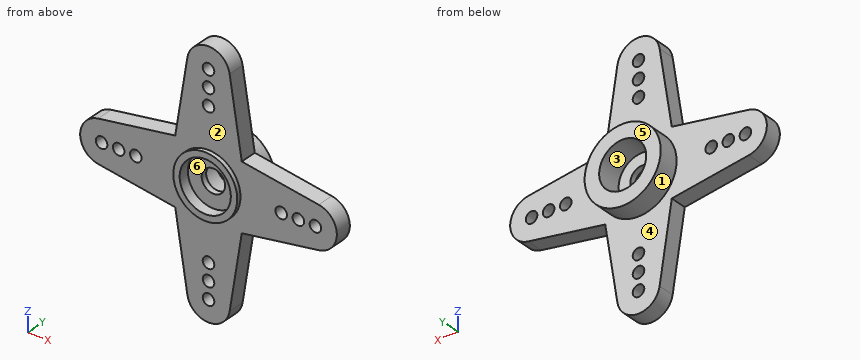
Autodesk Inventor part; units mm, degrees
ref_plane "YZ Plane" through (0, 0, 0) normal (1, 0, 0) x (0, 1, 0)
ref_plane "XZ Plane" through (0, 0, 0) normal (0, 1, 0) x (-1, 0, 0)
ref_plane "XY Plane" through (0, 0, 0) normal (0, 0, 1) x (1, 0, 0)
sketch "Sketch1" plane through (0, 0, 0) normal (0, 1, 0) x (-1, 0, 0)
  circle A0 centre (0, 0) radius 3.74
  circle A1 centre (0, 0) radius 4.45
  circle A2 centre (0, 0) radius 8.5
  circle A3 centre (0, 0) radius 10.5
  circle A4 centre (0, 0) radius 12.5
  circle A5 centre (12.5, 0) radius 2.5
  line L0 (0.6942, 4.3955) -> (12.89, 2.4694)
  line L1 (0.6942, -4.3955) -> (12.89, -2.4694)
  circle A6 centre (12.5, 0) radius 0.675
  circle A7 centre (10.5, -0.0001) radius 0.675
  circle A8 centre (8.5, 0.0004) radius 0.675
  line L2 (-4.3955, 0.6942) -> (-2.4694, 12.89)
  circle A9 centre (0, 12.5) radius 2.5
  circle A10 centre (0, 12.5) radius 0.675
  circle A11 centre (0.0001, 10.5) radius 0.675
  circle A12 centre (-0.0004, 8.5) radius 0.675
  line L3 (4.3955, 0.6942) -> (2.4694, 12.89)
  line L4 (-0.6942, -4.3955) -> (-12.89, -2.4694)
  circle A13 centre (-12.5, 0) radius 2.5
  circle A14 centre (-12.5, 0) radius 0.675
  circle A15 centre (-10.5, 0.0001) radius 0.675
  circle A16 centre (-8.5, -0.0004) radius 0.675
  line L5 (-0.6942, 4.3955) -> (-12.89, 2.4694)
  line L6 (4.3955, -0.6942) -> (2.4694, -12.89)
  circle A17 centre (0, -12.5) radius 2.5
  circle A18 centre (0, -12.5) radius 0.675
  circle A19 centre (-0.0001, -10.5) radius 0.675
  circle A20 centre (0.0004, -8.5) radius 0.675
  line L7 (-4.3955, -0.6942) -> (-2.4694, -12.89)
  point P0 (3.8907, 3.8907)
  point P1 (-3.8907, 3.8907)
  point P2 (-3.8907, -3.8907)
  point P3 (3.8907, -3.8907)
  dimension "d5" = 17
  dimension "d6" = 21
  dimension "d7" = 25
  dimension "d3" = 7.48
  dimension "d4" = 8.9
  dimension "d8" = 5
  dimension "d11" = 1.35
  dimension "d12" = 1.35
  dimension "d13" = 1.35
  dimension "d16" = 360
extrude "Extrusion1" add sketch "Sketch1" along normal blind 2 contours A1 L3 L0 A2 A8 L1 L6 | A1 L0 L3 | L6 L1 A1 | A1 L5 L2 A2 A12 L3 L0 | L1 L6 A2 A20 L7 L4 A1 | A1 L2 L5 | L0 A3 A5 A7 L1 A2 A8 | A2 A12 L2 A3 A9 A11 L3 | L4 L7 A1 | L6 A3 A17 A19 L7 A2 A20 | A1 L7 L4 A2 A16 L5 L2 | L0 A4 A5 A3 | A3 A9 A4 L3 | A3 A5 A4 L1 | L6 A4 A17 A3 | A2 A16 L4 A3 A13 A15 L5 | A5 A4 A6 A3 A7 | A3 A7 A5 | L0 A5 A4 | A9 A11 A3 | A3 A11 A9 A4 A10 | A4 A9 L3 | A5 A7 A3 | A4 A5 L1 | A17 A4 A18 A3 A19 | A3 A19 A17 | L6 A17 A4 | L2 A4 A9 A3 | A3 A13 A4 L5 | A5 A4 A6 | A4 A10 A9 | L4 A4 A13 A3 | A3 A17 A4 L7 | A17 A4 A18 | A3 A11 A9 | L2 A9 A4 | A13 A15 A3 | A3 A15 A13 A4 A14 | A4 A13 L5 | A3 A15 A13 | L4 A13 A4 | A17 A19 A3 | A4 A17 L7 | A4 A14 A13 picked at (10.283, 0.9379) picked at (0.938, 10.2831) picked at (10.2831, -0.938) picked at (0.9379, -10.283) picked at (-0.9379, 10.283) picked at (-10.2831, 0.938) picked at (-10.283, -0.9379) picked at (-0.938, -10.2831)
extrude "Extrusion2" add sketch "Sketch1" along normal blind 4.44 contours A1
ref_plane "Work Plane2" through (0, 1.44, 0) normal (0, 1, 0) x (1, 0, 0)
sketch "Sketch3" plane through (0, 1.44, 0) normal (0, 1, 0) x (1, 0, 0)
  circle A0 centre (0, 0) radius 1.37
  circle A1 centre (0, 0) radius 2.75
  circle A2 centre (0, 0) radius 2.99
  circle A3 centre (0, 0) radius 3.74
  dimension "d32" = 2.74
  dimension "d33" = 5.5
  dimension "d34" = 5.98
  dimension "d35" = 7.48
extrude "Extrusion6" add sketch "Sketch3" along normal blind 3 and the other way blind 1.94 contours A3
extrude "Extrusion7" add sketch "Sketch3" along normal blind 3 and the other way blind 0.69 contours A2
extrude "Extrusion8" add sketch "Sketch3" against normal blind 0.69 contours A1
properties part number "Standard Servo Horn - White Cross"
Can you work these out from the model? Positions are in its coordinate system, mm. Face numbers are marked on the shaded views. A direction names the side the tool comes from. Give positions to 0.01 mm unless a question says otherwise; leave off trailing zeros. Loops run counter-clockwise (first coordinate to the right, second up) from the corner with the lowest first, then second, coordinate; pieces in that order, holes last. Notation, with made-up numbers: M 80,35 L 138,35 A11 ccw 138,51 Z; hole C 34.5,-18 d3. An arc over 180 degrees is marked long. Use CSV: the item, a comma, the result in double quotes. Start each with the question number.
1. Imagine slicing it at A-A, the plane z = 10.5. Write out the boundary of the cut face in (x, y), plus the area to 3 significant figures.
2. Imagine slicing it at B-B, the plane x = 12.5. Write out the boundary of the cut face in (y, z) (3 decimals).
3. If we mould it in two halves opening along X, with no side actions, what happens to the marked faces 1, 2 and 3? For each: released by +X, released by -X, zero draft, split by the parting line, or undercut.
4. For P1, Ø1.8, axis at x = 0, z = -12.5, coming from the -Y side; P2, Ø1.8, axis at x = 0, z = 8.5, coming from the +Y side; P3, Ø9, axis at x = -3.5, z = 6, coming from the +Y side, each with a flat end and sliding along its axis, tell me the tip position at first contact or that it passes through.
5. Imagine slicing it at D-D, the plane x = 0. Count the separate pieces of the cut face and the enclosed holes in it, plus the area to 3 significant figures.
6. On a 3-axis mill with a long thin cutter (end or side, diameter ignored), from which of +Z, -Z, +X, -X, +Y, -Y can I reach the whole of each face in a straight line? I mean the marked faces 4, 5 and 6. Say none if no direction works.
7. If I drill on L1, parallel to Y at x = -9.75, z = 1.25; L2, parallel to X at y = 1.4, z = -10.5; L3, parallel to Z at x = 0, y = 2.5, over which ranges is the centre line in solid material (lowest first)?
8. Imagine slicing it at C-C, the plane y = 2.9. Write out the boundary of the cut face in (x, z).
Response values:
1,outline,"M -2.85,0 L -0.68,0 L -0.68,2 L -2.85,2 Z; M 0.67,0 L 2.85,0 L 2.85,2 L 0.67,2 Z"
1,area,"8.69 mm^2"
2,outline,"M 0,-2.531 L 2,-2.531 L 2,-0.675 L 0,-0.675 Z; M 0,0.675 L 2,0.675 L 2,2.531 L 0,2.531 Z"
3,face 1,"split by the parting line"
3,face 2,"zero draft"
3,face 3,"undercut"
4,P1,"y = 0"
4,P2,"y = 2"
4,P3,"y = 4.44"
5,separate pieces,"8"
5,enclosed holes,"0"
5,area,"43.4 mm^2"
6,face 4,"+Y"
6,face 5,"+Z, -Z, +X, -X, +Y"
6,face 6,"-Y"
7,L1,"0 to 2"
7,L2,"-2.85 to -0.67, 0.68 to 2.85"
7,L3,"-4.45 to -2.75, 2.75 to 4.45"
8,outline,"C 0,0 d8.9; hole C 0,0 d5.5"
